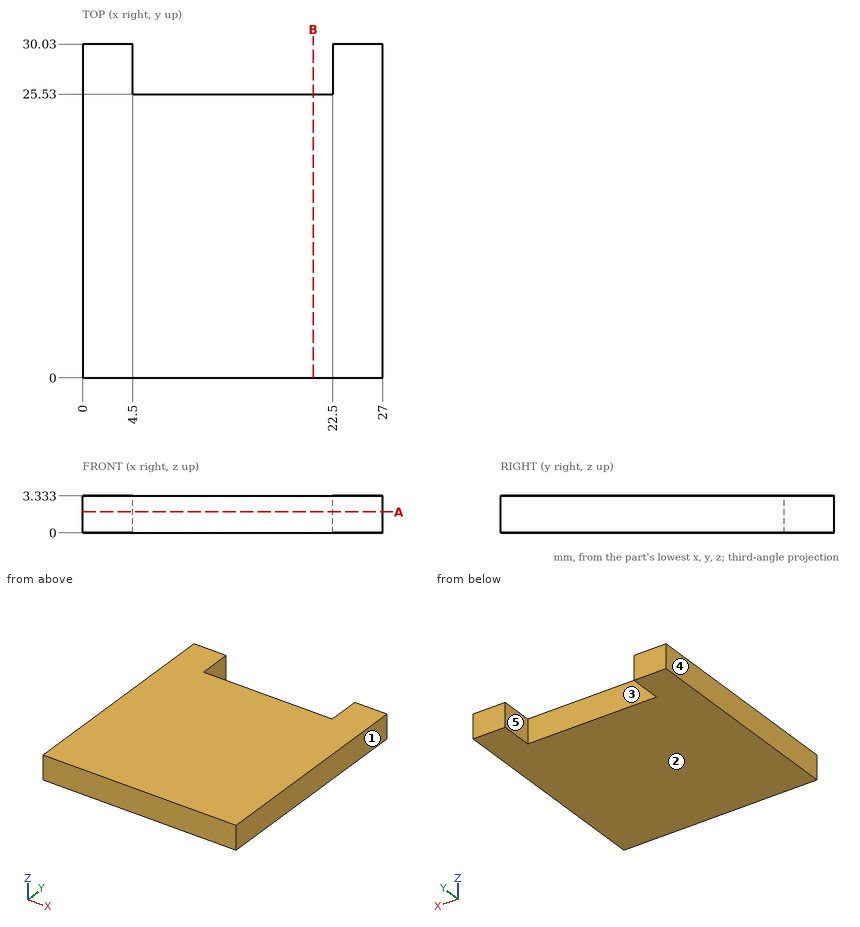
Geometry check sheet. Reference: drawing and pictorial views, mm from the part's lowest x, y, z. A direction names the side the tool comes from. Give positions to 0.01 mm unless a question says otherwise; leave off trailing zeros. Write each loop counter-clockwise with the first axis right and the second up, starting at its lowest first coordinate (ties: lowest second). Pieces come first, ordered by that corner, then holes. Notation, with made-up numbers: (15, 38) -> (24, 38) arc R30 ccw to (24, 72) -> close; hole circle Ø8 at (2, -18). An arc over 180 degrees is marked (long way). One line per item, written item: value. Start each with the question number.
Item 1: Material ranges on probe 1 along X at (y, z) = (28, 2.65); probe 2 along Y at (x, z) = (19.5, 2.7), recorded low to high. Write a range as from..to.
Item 2: Tool access check on the marked faces 4 and 5. Record the directions out of +Z, -Z, +X, -X, +Y, -Y that give a thin tool (end or side, any length) a straight path to the whole face; none if there is none.
Item 3: Section check A-A on z = 1.9. Record the cut outline in (x, y).
Item 4: Gauge pin test, flat ends, axial feed: pin 1 (12 mm diameter, centred on x = 9, y = 13, fed in from -Z); pin 2 (1.7 mm diameter, centred on x = 14.5, z = 2, fed in from +Y). Record the tip position at first contact, or that the pin passes through.
Item 5: Section check B-B on x = 20.75. Record the cut outline in (y, z), then the cut area to 3 significant figures.
Item 6: Draft check along X on the marked faces 1, 2 and 3. Enter one of: +X half, -X half, draft (parallel to the pull), parting line (faces both ways), or undercut.
Results list:
1. probe 1: 0..4.5, 22.5..27
1. probe 2: 0..25.53
2. face 4: +Z, -Z, -X, +Y, -Y
2. face 5: +Z, -Z, +Y
3. outline: (0, 0) -> (27, 0) -> (27, 30.03) -> (22.5, 30.03) -> (22.5, 25.53) -> (4.5, 25.53) -> (4.5, 30.03) -> (0, 30.03) -> close
4. pin 1: z = 0
4. pin 2: y = 25.53
5. outline: (0, 0) -> (25.53, 0) -> (25.53, 3.33) -> (0, 3.33) -> close
5. area: 85.1 mm²
6. face 1: +X half
6. face 2: draft
6. face 3: undercut
